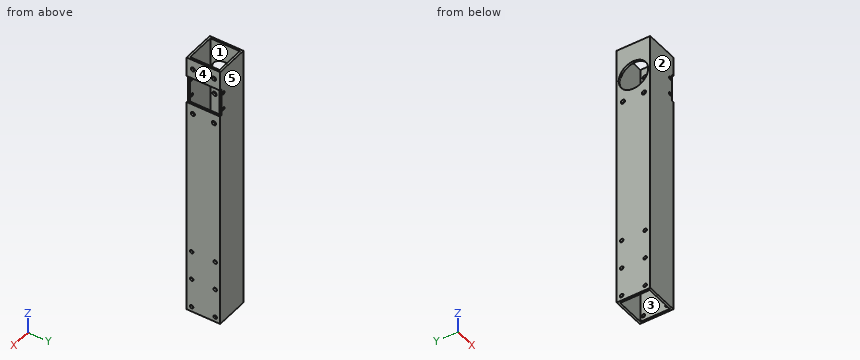
Autodesk Inventor part; units mm, degrees
ref_plane "YZ Plane" through (0, 0, 0) normal (1, 0, 0) x (0, 1, 0)
ref_plane "XZ Plane" through (0, 0, 0) normal (0, 1, 0) x (-1, 0, 0)
ref_plane "XY Plane" through (0, 0, 0) normal (0, 0, 1) x (1, 0, 0)
sketch "Sketch1" plane through (0, 0, 0) normal (0, 0, 1) x (1, 0, 0)
  line L0 (-35.56, 0) -> (35.56, 0) construction
  line L1 (0, -35.56) -> (0, 35.56) construction
  line L2 (-25.4, 25.4) -> (25.4, 25.4)
  line L3 (25.4, 25.4) -> (25.4, -25.4)
  line L4 (25.4, -25.4) -> (-25.4, -25.4)
  line L5 (-25.4, -25.4) -> (-25.4, 25.4)
  line L6 (-22.225, 22.225) -> (22.225, 22.225)
  line L7 (22.225, 22.225) -> (22.225, -22.225)
  line L8 (22.225, -22.225) -> (-22.225, -22.225)
  line L9 (-22.225, -22.225) -> (-22.225, 22.225)
  point P0 (0, 0)
  point P1 (-25.4, 0)
  point P2 (0, 25.4)
  point P3 (-22.225, 0)
  point P4 (0, 22.225)
  dimension "d0" = 50.8
  dimension "d1" = 3.175
extrude "Extrusion1" add sketch "Sketch1" along normal mid plane 406.4
sketch "Sketch2" plane through (25.4, -25.4, 203.2) normal (1, 0, 0) x (0, 0, -1)
  line L0 (542.6964, 25.4) -> (-90.4494, 25.4) construction
  line L1 (203.2, -10.16) -> (203.2, 60.96) construction
  line L2 (309.88, 7.62) -> (398.78, 7.62) construction
  line L3 (398.78, 7.62) -> (398.78, 43.18) construction
  line L4 (398.78, 43.18) -> (309.88, 43.18) construction
  line L5 (309.88, 43.18) -> (309.88, 7.62) construction
  circle A0 centre (309.88, 43.18) radius 2.667
  circle A1 centre (309.88, 7.62) radius 2.667
  circle A2 centre (354.33, 7.62) radius 2.667
  circle A3 centre (398.78, 7.62) radius 2.667
  circle A4 centre (398.78, 43.18) radius 2.667
  circle A5 centre (354.33, 43.18) radius 2.667
  line L6 (406.4, 50.8) -> (406.4, 0) construction
  point P0 (203.2, 25.4)
  point P1 (398.78, 25.4)
  dimension "d4" = 5.334
  dimension "d5" = 7.62
  dimension "d6" = 88.9
  dimension "d7" = 17.78
extrude "Extrusion2" cut sketch "Sketch2" against normal through all
sketch "Sketch10" plane through (25.4, -25.4, 203.2) normal (1, 0, 0) x (0, 0, -1)
  line L0 (487.68, 25.4) -> (-81.28, 25.4) construction
  circle A0 centre (398.78, 43.18) radius 2.667 construction
  circle A1 centre (354.33, 7.62) radius 2.667 construction
  circle A2 centre (309.88, 43.18) radius 2.667 construction
  circle A3 centre (309.88, 7.62) radius 2.667 construction
  circle A4 centre (398.78, 7.62) radius 2.667 construction
  circle A5 centre (354.33, 43.18) radius 2.667 construction
  line L1 (0, 50.8) -> (406.4, 50.8) construction
  line L2 (0, 0) -> (0, 50.8) construction
  line L3 (0, 0) -> (406.4, 0) construction
  line L4 (406.4, 50.8) -> (406.4, 0) construction
  line L5 (29.7942, 50.8) -> (71.8058, 50.8)
  line L6 (71.8058, 50.8) -> (71.8058, 0)
  line L7 (71.8058, 0) -> (29.7942, 0)
  line L8 (29.7942, 0) -> (29.7942, 50.8)
  line L9 (29.7942, 50.8) -> (71.8058, 0) construction
  point P0 (203.2, 25.4)
  point P1 (50.8, 25.4)
  point P2 (29.7942, 25.4)
  dimension "d47" = 50.8
  dimension "d48" = 42.0116
  dimension "d49" = 50.8
extrude "Extrusion9" cut sketch "Sketch10" against normal blind 3.175
sketch "Sketch11" plane through (-25.4, 25.4, -203.2) normal (0, 1, 0) x (1, 0, 0)
  circle A0 centre (43.7, -368.3) radius 2.0193 construction
  circle A1 centre (43.7, -342.9) radius 2.0193 construction
  circle A2 centre (43.7, -342.9) radius 2.413
  circle A3 centre (43.7, -368.3) radius 2.413
  point P0 (25.4, -203.2)
  dimension "d73" = 4.826
sketch "Sketch12" plane through (-25.4, -25.4, 203.2) normal (-1, 0, 0) x (0, 0, 1)
  line L0 (-487.68, 25.4) -> (81.28, 25.4) construction
  circle A0 centre (-398.78, 43.18) radius 2.667 construction
  circle A1 centre (-354.33, 7.62) radius 2.667 construction
  circle A2 centre (-309.88, 43.18) radius 2.667 construction
  circle A3 centre (-309.88, 7.62) radius 2.667 construction
  circle A4 centre (-398.78, 7.62) radius 2.667 construction
  circle A5 centre (-354.33, 43.18) radius 2.667 construction
  line L1 (0, 0) -> (-406.4, 0) construction
  line L2 (0, 50.8) -> (0, 0) construction
  line L3 (-406.4, 50.8) -> (0, 50.8) construction
  line L4 (-406.4, 0) -> (-406.4, 50.8) construction
  circle A6 centre (-50.8, 25.4) radius 22.225
  point P0 (-203.2, 25.4)
  dimension "d54" = 50.8
  dimension "d55" = 44.45
extrude "Extrusion11" cut sketch "Sketch12" against normal blind 3.175
sketch "Sketch14" plane through (22.225, -22.225, -203.2) normal (-1, 0, 0) x (0, 0, 1)
  line L0 (-81.28, 22.225) -> (487.68, 22.225) construction
  circle A0 centre (355.6, 22.225) radius 22.225 construction
  line L1 (355.6, 0) -> (355.6, 44.45) construction
  line L2 (391.5029, 6.35) -> (319.6971, 6.35) construction
  line L3 (319.6971, 6.35) -> (319.6971, 38.1) construction
  line L4 (319.6971, 38.1) -> (391.5029, 38.1) construction
  line L5 (391.5029, 38.1) -> (391.5029, 6.35) construction
  circle A1 centre (391.5029, 6.35) radius 3.175
  circle A2 centre (391.5029, 38.1) radius 3.175
  circle A3 centre (319.6971, 6.35) radius 3.175
  circle A4 centre (319.6971, 38.1) radius 3.175
  line L6 (406.4, 0) -> (376.6058, 0)
  point P0 (203.2, 22.225)
  point P1 (391.5029, 22.225)
  point P2 (391.5029, 0)
  dimension "d67" = 6.35
  dimension "d68" = 31.75
extrude "Extrusion12" cut sketch "Sketch14" against normal through all
sketch "Sketch15" plane through (-25.4, -25.4, 203.2) normal (-1, 0, 0) x (0, 0, 1)
  circle A0 centre (-86.7029, 9.525) radius 3.175
  circle A1 centre (-86.7029, 41.275) radius 3.175
  point P0 (-203.2, 25.4)
extrude "Extrusion13" cut sketch "Sketch15" against normal up to next
extrude "Extrusion14" cut sketch "Sketch11" against normal through all
properties part number "Arm 18 inch" material "Aluminum 6061"
Verification items for the finished model (mm, model axes). Face numbers are marked on the shaded views. A direction names the side the tool comes from. Coordinates: 2 decimals unless noted, no trailing zeros. Loops run counter-clockwise (first coordinate to the right, second up) from the corner with the lowest first, then second, coordinate; pieces in that order, holes last. Notation, with made-up numbers: (29, -1.75) -> (47, -1.75) arc R24 cw to (47, 32.25) -> close; hole circle Ø5 at (57.25, 9). An arc over 180 degrees is marked (long way). Answer as a JSON object with one key per item and string values. Group by question number.
Item 1: Scan lines: probe 1 along Z at (x, y) = (18.3, 24.4); probe 2 along Y at (x, z) = (-24.7, -106.68); probe 3 along Y at (x, z) = (24, -195). Record each from-to range of solid material in increasing order.
Item 2: Mould release check, pull along X, two halves, no side actions. Record for the marked faces 3, 4 and 5: +X half, -X half, draft (parallel to the pull), parting line (faces both ways), or undercut.
Item 3: Sectioned sample at B-B on x = -1.5. Record the boundary of the cut face in (y, z) (3 decimals), plus the area to 3 significant figures.
Item 4: Tool access check on the marked faces 1 and 2. Record the directions out of +Z, -Z, +X, -X, +Y, -Y that give a thin tool (end or side, any length) a straight path to the whole face; none if there is none.
Item 5: Sectioned sample at A-A on y = 0. Record the boundary of the cut face in (x, z) (3 decimals), plus the area to 3 significant figures.
Item 6: Sectioned sample at C-C on z = 57. Record the boundary of the cut face in (x, y) (3 decimals).
Evaluation:
{
 "1": {"probe 1": "z = -203.2 to 137.29, 142.11 to 162.69, 167.51 to 203.2", "probe 2": "y = -25.4 to -20.45, -15.11 to 15.11, 20.45 to 25.4", "probe 3": "y = -25.4 to -20.38, -15.18 to 15.18, 20.38 to 25.4"},
 "2": {"face 3": "undercut", "face 4": "+X half", "face 5": "draft"},
 "3": {"outline": "(-25.4, -203.2) -> (-22.225, -203.2) -> (-22.225, 203.2) -> (-25.4, 203.2) -> close; (22.225, -203.2) -> (25.4, -203.2) -> (25.4, 203.2) -> (22.225, 203.2) -> close", "area": "2,580 mm²"},
 "4": {"face 1": "+Z, -Z", "face 2": "+Z, -Z, +X, -X, -Y"},
 "5": {"outline": "(-25.4, -203.2) -> (-22.225, -203.2) -> (-22.225, 130.175) -> (-25.4, 130.175) -> close; (-25.4, 174.625) -> (-22.225, 174.625) -> (-22.225, 203.2) -> (-25.4, 203.2) -> close; (22.225, -203.2) -> (25.4, -203.2) -> (25.4, 131.394) -> (22.225, 131.394) -> close; (22.225, 173.406) -> (25.4, 173.406) -> (25.4, 203.2) -> (22.225, 203.2) -> close", "area": "2,310 mm²"},
 "6": {"outline": "(-25.4, -25.4) -> (25.4, -25.4) -> (25.4, 25.4) -> (-25.4, 25.4) -> close; hole (-22.225, -22.225) -> (22.225, -22.225) -> (22.225, 22.225) -> (-22.225, 22.225) -> close"}
}
